Verification items for this drawing (mm, ordinates from the low corner). A direction names the side the tool comes from. Round coordinates to 2 decimals unless told otherwise and drop trailing zeros. Loops run counter-clockwise (first coordinate to the right, second up) from the corner with the lowest first, then second, coordinate; pieces in that order, holes last. Notation, with made-up numbers: M 17,-7 L 57,-7 A34 cw 57,29 Z; hole C 49.5,13 d9. An arc over 180 degrees is marked long. Answer as CSV lines item,"result".
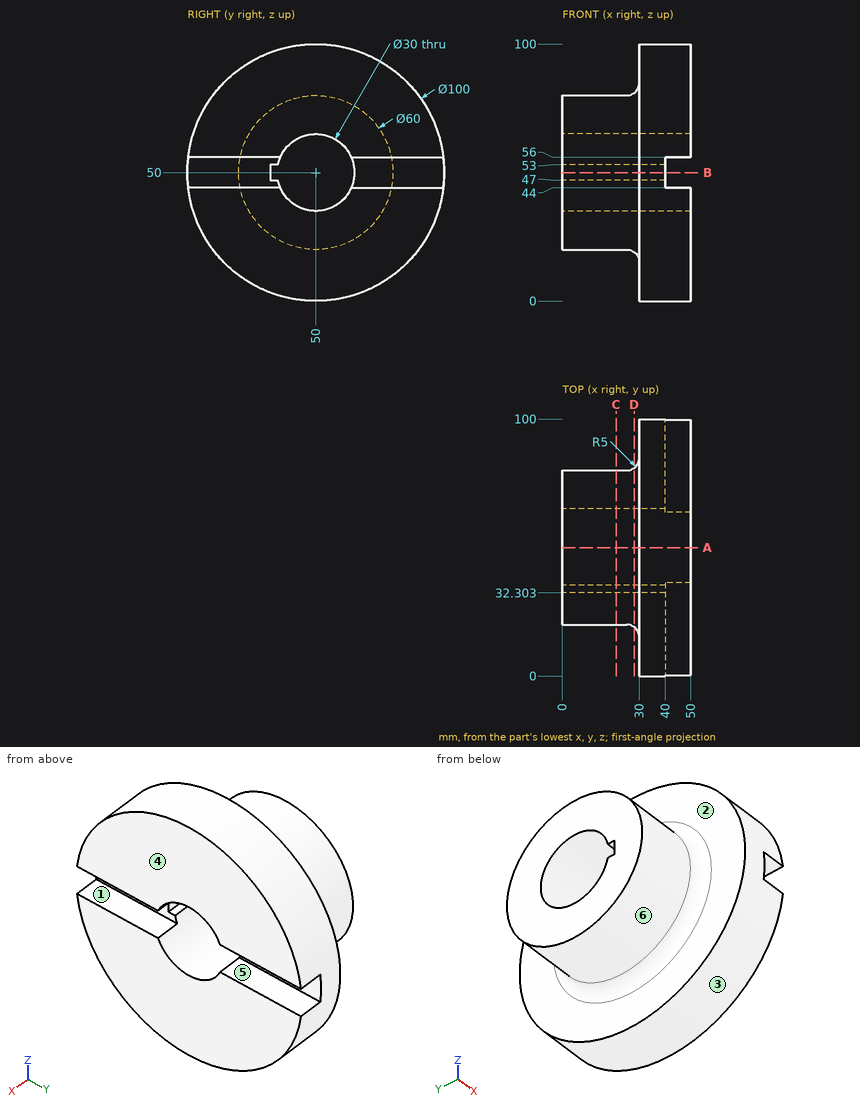
1) Section check C-C (x = 21). Record the cut outline in (y, z), plus the area to 3 significant figures.
Here are the results:
outline,"C 50,50 d60; hole M 32.3,47 L 35.3,47 A15 ccw long 35.3,53 L 32.3,53 Z"
area,"2,100 mm^2"
2) Material ranges on probe 1 along Y at (x, z) = (33.5, 50); probe 2 along Z at (x, y) = (22, 50); probe 3 along X at (y, z) = (9, 32.5), recorded low to high.
Here are the results:
probe 1,"y = 0 to 32.3, 65 to 100"
probe 2,"z = 20 to 35, 65 to 80"
probe 3,"x = 30 to 50"
3) Go/stop test with flat-tipped pins: pin 1 (2.5 mm diameter, centred on x = 24.5, y = 33.5, fed in from -Z) (3 decimals); pin 2 (5 mm diameter, centred on x = 46.5, y = 23.5, fed in from -Z); pin 3 (5 mm diameter, centred on x = 8, z = 26, fed in from -Y). Record where each tip stops, or that it passes through.
Here are the results:
pin 1,"stops at z = 24.165"
pin 2,"stops at z = 6.14"
pin 3,"stops at y = 29.08"
4) Set-up check for the marked faces 1, 2 and 3: record each of +Z, -Z, +X, -X, +Y, -Y from which the full face is reachable in a straight line by a thin tool's end or side.
Here are the results:
face 1,"+X, +Y, -Y"
face 2,"-X"
face 3,"+X, -X"
5) Section check A-A (y = 50). Record the cut outline in (x, z).
Here are the results:
outline,"M 0,20 L 25,20 A5 cw 30,15 L 30,0 L 50,0 L 50,35 L 0,35 Z; M 0,65 L 50,65 L 50,100 L 30,100 L 30,85 A5 cw 25,80 L 0,80 Z"
6) Draft check along Z on the marked faces 4, 5 and 6. Enter one of: +Z half, -Z half, draft (parallel to the pull), parting line (faces both ways), or undercut.
Here are the results:
face 4,"draft"
face 5,"undercut"
face 6,"parting line"
7) Section check B-B (z = 50). Record the cut outline in (x, y), plus the area to 3 significant figures.
Here are the results:
outline,"M 0,20 L 25,20 A5 cw 30,15 L 30,0 L 40,0 L 40,32.3 L 0,32.3 Z; M 0,65 L 40,65 L 40,100 L 30,100 L 30,85 A5 cw 25,80 L 0,80 Z"
area,"1,500 mm^2"
8) Section check D-D (x = 28). Record the cut outline in (y, z).
Here are the results:
outline,"C 50,50 d62; hole M 32.3,47 L 35.3,47 A15 ccw long 35.3,53 L 32.3,53 Z"
